For this review, take the finished solid that the model builds, in its own axes (mm). A direction names the side the tool comes from. Give positions to 0.01 mm unless a question says otherwise; leave off trailing zeros. Write each loop counter-clockwise with the first axis right and the second up, starting at its lowest first coordinate (ties: lowest second). Pieces come first, ordered by that corner, then holes. Notation, with made-up numbers: (6, 42.25) -> (46, 42.25) arc R23 ccw to (46, 58.25) -> close; hole circle Ø3 at (-37, -25.5). An arc over 180 degrees is marked (long way). Write item = value, one per line.
Autodesk Inventor part; units mm, degrees
ref_plane "YZ Plane" through (0, 0, 0) normal (1, 0, 0) x (0, 1, 0)
ref_plane "XZ Plane" through (0, 0, 0) normal (0, 1, 0) x (-1, 0, 0)
ref_plane "XY Plane" through (0, 0, 0) normal (0, 0, 1) x (1, 0, 0)
sketch "Sketch1" plane through (0, 0, 0) normal (0, 0, 1) x (1, 0, 0)
  line L0 (-28.9, -19.5) -> (28.9, -19.5)
  line L1 (28.9, -19.5) -> (28.9, 19.5)
  line L2 (28.9, 19.5) -> (-28.9, 19.5)
  line L3 (-28.9, 19.5) -> (-28.9, -19.5)
  line L4 (-28.9, -19.5) -> (28.9, 19.5) construction
  line L5 (28.9, -19.5) -> (-28.9, 19.5) construction
  point P0 (0, 0)
  dimension "d0" = 57.8
  dimension "d1" = 39
extrude "Extrusion1" add sketch "Sketch1" along normal blind 9.61
sketch "Sketch2" plane through (0, 0, 0) normal (0, 0, -1) x (-1, 0, 0)
  circle A0 centre (-21.6, -15.1) radius 0.8
  line L0 (55.7735, 0) -> (-51.4211, 0) construction
  line L1 (0, -27.3) -> (0, 27.3) construction
  line L2 (28.9, -19.5) -> (-28.9, -19.5)
  line L3 (-28.9, -19.5) -> (-28.9, 19.5)
  circle A1 centre (21.6, -15.1) radius 0.8
  line L4 (-36.1076, -0.7) -> (40.46, -0.7) construction
  circle A2 centre (-21.6, 13.7) radius 0.8
  circle A3 centre (21.6, 13.7) radius 0.8
  line L5 (-28.9, 19.5) -> (28.9, 19.5)
  point P0 (0, 0)
  dimension "d4" = 1.6
  dimension "d5" = 4.4
  dimension "d6" = 7.3
  dimension "d7" = 5.8
extrude "Extrusion2" cut sketch "Sketch2" against normal through all
sketch "Sketch3" plane through (0, 0, 0) normal (0, 0, -1) x (-1, 0, 0)
  line L0 (-28.9, 19.5) -> (28.9, 19.5) construction
  line L1 (28.9, -19.5) -> (-28.9, -19.5) construction
  line L2 (-28.9, -19.5) -> (-28.9, 19.5)
  line L3 (-26.9, 19.5) -> (-26.9, -0.4)
  line L4 (-24.9, -2.4) -> (-19.85, -2.4)
  line L5 (-17.85, -4.4) -> (-17.85, -11.3)
  line L6 (-19.85, -13.3) -> (-24.9, -13.3)
  line L7 (-26.9, -15.3) -> (-26.9, -19.5)
  line L8 (-28.9, 19.5) -> (28.9, 19.5)
  line L9 (-26.9, 19.5) -> (-28.9, 19.5)
  line L10 (-28.9, 19.5) -> (-28.9, -19.5)
  arc A0 (-26.9, -0.4) -> (-24.9, -2.4) centre (-24.9, -0.4) ccw
  arc A1 (-17.85, -4.4) -> (-19.85, -2.4) centre (-19.85, -4.4) ccw
  arc A2 (-19.85, -13.3) -> (-17.85, -11.3) centre (-19.85, -11.3) ccw
  arc A3 (-24.9, -13.3) -> (-26.9, -15.3) centre (-24.9, -15.3) ccw
  line L11 (-28.9, 19.5) -> (-26.9, 19.5)
  line L12 (-28.9, -19.5) -> (-28.9, 19.5)
  line L13 (-28.9, -19.5) -> (-26.9, -19.5)
  line L14 (0, -27.3) -> (0, 27.3)
  line L15 (28.9, -19.5) -> (28.9, 19.5)
  line L16 (26.9, 19.5) -> (26.9, -0.4)
  line L17 (24.9, -2.4) -> (19.85, -2.4)
  line L18 (17.85, -4.4) -> (17.85, -11.3)
  line L19 (19.85, -13.3) -> (24.9, -13.3)
  line L20 (26.9, -15.3) -> (26.9, -19.5)
  line L21 (26.9, 19.5) -> (28.9, 19.5)
  line L22 (28.9, 19.5) -> (28.9, -19.5)
  arc A4 (24.9, -2.4) -> (26.9, -0.4) centre (24.9, -0.4) ccw
  arc A5 (19.85, -2.4) -> (17.85, -4.4) centre (19.85, -4.4) ccw
  arc A6 (17.85, -11.3) -> (19.85, -13.3) centre (19.85, -11.3) ccw
  arc A7 (26.9, -15.3) -> (24.9, -13.3) centre (24.9, -15.3) ccw
  line L23 (28.9, 19.5) -> (26.9, 19.5)
  line L24 (28.9, -19.5) -> (28.9, 19.5)
  line L25 (28.9, -19.5) -> (26.9, -19.5)
  point P0 (0, 0)
  point P1 (-26.9, -13.3)
  point P2 (26.9, -13.3)
  dimension "d10" = 6.2
  dimension "d11" = 21.9
  dimension "d12" = 11.05
  dimension "d13" = 2
  dimension "d14" = 2
extrude "Extrusion3" cut sketch "Sketch3" against normal blind 1.2
fillet "Fillet1" radius 2 4 edges at (-28.9, 19.5, 5.405) (28.9, 19.5, 5.405) (28.9, -19.5, 5.405) (-28.9, -19.5, 5.405)
properties part number "ThermalConductivityBlock_NX"
(1) To check wall thickness, follow probe 1 along Y at (x, z) = (21.6, 3); probe 2 along X at (y, z) = (13.5, 7); probe 3 along X at (y, z) = (4.5, 1). State the ranges of each line that lie inside material, in increasing order.
Answers below:
probe_1 = -19.5 to -15.9, -14.3 to 12.9, 14.5 to 19.5
probe_2 = -28.9 to -22.37, -20.83 to 20.83, 22.37 to 28.9
probe_3 = -26.9 to 26.9
(2) Take a section at A-A (x = 21.6). Write out the cut boundary in (y, z), plus the area to 3 significant figures.
Answers below:
outline = (-19.5, 0) -> (-15.9, 0) -> (-15.9, 9.61) -> (-19.5, 9.61) -> close; (-14.3, 0) -> (-13.3, 0) -> (-13.3, 1.2) -> (-2.4, 1.2) -> (-2.4, 0) -> (12.9, 0) -> (12.9, 9.61) -> (-14.3, 9.61) -> close; (14.5, 0) -> (19.5, 0) -> (19.5, 9.61) -> (14.5, 9.61) -> close
area = 331 mm^2
(3) The part is to be moulded in two halves that separate along Y. For faces 5 (the face through (26.9, -17, 1)), 6 (the face through (-20.8, -15.1, 4.7)), 7 (the face through (-28.33, -18.9, 5.46)), say which applies: released by +Y, released by -Y, zero draft, split by the parting line, or undercut.
Answers below:
face_5 = zero draft
face_6 = undercut
face_7 = released by -Y
(4) Tool access review of faces 1 (the face through (0, 0, 9.61)), 2 (the face through (26.9, 10, 1)), 3 (the face through (-17.85, -8, 1)), 4 (the face through (17.85, -8, 1)): name each direction out of +Z, -Z, +X, -X, +Y, -Y from which nothing blocks a thin tool from reaching the whole face with its end or side.
Answers below:
face_1 = +Z, +X, -X, +Y, -Y
face_2 = -Z, +X, +Y, -Y
face_3 = -Z, -X
face_4 = -Z, +X
(5) Take a section at B-B (y = 13.7). Write out the cut boundary in (x, z).
Answers below:
outline = (-28.9, 1.2) -> (-26.9, 1.2) -> (-26.9, 0) -> (-22.4, 0) -> (-22.4, 9.61) -> (-28.9, 9.61) -> close; (-20.8, 0) -> (20.8, 0) -> (20.8, 9.61) -> (-20.8, 9.61) -> close; (22.4, 0) -> (26.9, 0) -> (26.9, 1.2) -> (28.9, 1.2) -> (28.9, 9.61) -> (22.4, 9.61) -> close
(6) For pin 1 (1 mm diameter, centred on y = 10.5, z = 0.5, fed in from +X); pin 2 (1 mm diameter, centred on y = -18, z = 0.5, fed in from -X), all flat-tipped, find the tip position at first contact; note any pin that passes through.
Answers below:
pin_1 = 26.9
pin_2 = -26.9
